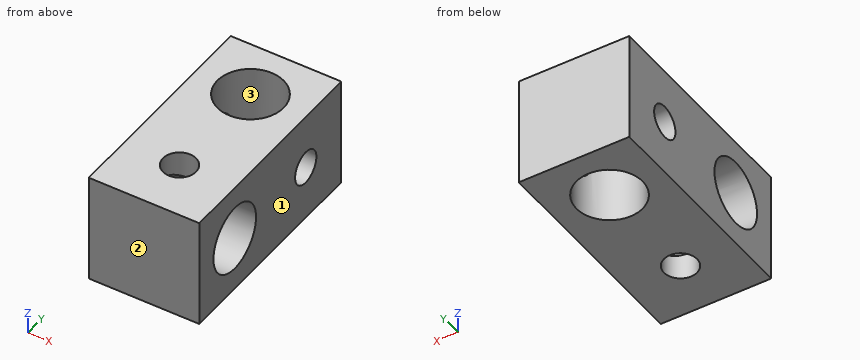
from build123d import *

# Parameters (mm, degrees)
F0_W     = 10
F0_H     = 20
F0_R     = 1.5
F0_R_2   = 3
F1_DEPTH = 10
F2_R     = 3
F2_R_2   = 1.5
F3_DEPTH = 25


with BuildPart() as f1:
    # F0 (on Top) → F1 (new body)
    with BuildSketch(Plane.XY):
        Rectangle(F0_W, F0_H)
        with Locations((0, -5)):
            Circle(F0_R, mode=Mode.SUBTRACT)
        with Locations((0, 5)):
            Circle(F0_R_2, mode=Mode.SUBTRACT)
    extrude(amount=F1_DEPTH)

    # F2 (on face) → F3 (cut)
    with BuildSketch(Plane(origin=(-5, 0, 0), x_dir=(0, -1, 0), z_dir=(-1, 0, 0))):
        with Locations((5, 5)):
            Circle(F2_R)
        with Locations((-5, 5)):
            Circle(F2_R_2)
    extrude(amount=-F3_DEPTH, mode=Mode.SUBTRACT)


solid = f1.part
Verification items for the finished model (mm, model axes). Face numbers are marked on the shaded views. Coordinates: 2 decimals unless noted, no trailing zeros. Order: outer loops, then holes, each group sorted by start corner. A loop starts at its lowest first (then second) coordinate and runs counter-clockwise, first axis right, second up. Notation, with made-up numbers: M 0.5,15.5 L 12.5,15.5 A10 cw 12.5,26.5 Z; hole C 8.25,-27 d7. An arc over 180 degrees is marked long. One line per item, written item: value. Start each with the question number.
Item 1: Sectioned sample at B-B on y = -5. Record the cut outline in (x, z).
Item 2: Sectioned sample at D-D on x = -2.25. Record the cut outline in (y, z), then the cut area to 3 significant figures.
Item 3: Sectioned sample at A-A on x = 0. Record the cut outline in (y, z), then the cut area to 3 significant figures.
Item 4: Mould release check, pull along Y, two halves, no side actions. Record for the marked faces 1, 2 and 3: pulls with the +Y half, pulls with the -Y half, needs draft (parallel to the pull), parting line crosses it, or undercut.
Item 5: Sectioned sample at C-C on z = 5. Record the cut outline in (x, y), then the cut area to 3 significant figures.
Item 6: Thickness scan on probe 1 along Z at (x, y) = (-3.5, 5); probe 2 along Y at (x, z) = (0.5, 7.5); probe 3 along X at (y, z) = (5, 7). Record the ranges inside material, lowest first.
Calculated:
1. outline: M -5,0 L -1.5,0 L -1.5,2 L -5,2 Z; M -5,8 L -1.5,8 L -1.5,10 L -5,10 Z; M 1.5,0 L 5,0 L 5,2 L 1.5,2 Z; M 1.5,8 L 5,8 L 5,10 L 1.5,10 Z
2. outline: M -10,0 L 3.02,0 L 3.02,10 L -10,10 Z; M 6.98,0 L 10,0 L 10,10 L 6.98,10 Z; hole C -5,5 d6
2. area: 132 mm^2
3. outline: M -10,0 L -6.5,0 L -6.5,2.4 A3 cw -6.5,7.6 L -6.5,10 L -10,10 Z; M -3.5,0 L 2,0 L 2,10 L -3.5,10 L -3.5,7.6 A3 cw -3.5,2.4 Z; M 8,0 L 10,0 L 10,10 L 8,10 Z
3. area: 98.9 mm^2
4. face 1: needs draft
4. face 2: pulls with the -Y half
4. face 3: undercut
5. outline: M -5,-10 L 5,-10 L 5,-8 L -5,-8 Z; M -5,-2 L 5,-2 L 5,3.5 L 2.6,3.5 A3 cw -2.6,3.5 L -5,3.5 Z; M -5,6.5 L -2.6,6.5 A3 cw 2.6,6.5 L 5,6.5 L 5,10 L -5,10 Z
5. area: 98.9 mm^2
6. probe 1: 0 to 3.5, 6.5 to 10
6. probe 2: -10 to -6.66, -3.34 to 2.04, 7.96 to 10
6. probe 3: -5 to -3, 3 to 5
